Autodesk Inventor part; units mm, degrees
ref_plane "YZ Plane" through (0, 0, 0) normal (1, 0, 0) x (0, 1, 0)
ref_plane "XZ Plane" through (0, 0, 0) normal (0, 1, 0) x (-1, 0, 0)
ref_plane "XY Plane" through (0, 0, 0) normal (0, 0, 1) x (1, 0, 0)
sketch "Boceto1" plane through (0, 0, 0) normal (0, 1, 0) x (-1, 0, 0)
  line L0 (12.5, 6.25) -> (-12.5, 6.25)
  line L1 (-12.5, 6.25) -> (-12.5, -6.25)
  line L2 (-12.5, -6.25) -> (12.5, -6.25)
  line L3 (12.5, -6.25) -> (12.5, 6.25)
  line L4 (10.5, 4.25) -> (-10.5, 4.25)
  line L5 (-10.5, 4.25) -> (-10.5, -4.25)
  line L6 (-10.5, -4.25) -> (10.5, -4.25)
  line L7 (10.5, -4.25) -> (10.5, 4.25)
  point P0 (0, 0)
  point P1 (12.5, 0)
  point P2 (0, -6.25)
  point P3 (10.5, 0)
  point P4 (0, 4.25)
  dimension "d3" = 25
  dimension "d4" = 12.5
  dimension "d6" = 2
  dimension "d7" = 2
sketch "Boceto2" plane through (0, 0, 0) normal (0, 0, 1) x (1, 0, 0)
  line L0 (0, 0) -> (-62.7506, -84.1864)
  line L1 (0, 0) -> (0, -34.6116) construction
  dimension "d2" = 36.7
  dimension "d5" = 105
sweep "Barrido1" add profiles "Boceto1" path "Boceto2"
sketch "Boceto3" plane through (-12.5, 0, 6.25) normal (0, 0, 1) x (1, 0, 0)
  line L0 (0, 0) -> (25, 0)
  line L1 (0, 0) -> (-62.7506, -84.1864)
  line L2 (-37.7506, -84.1864) -> (-62.7506, -84.1864)
  line L3 (25, 0) -> (-37.7506, -84.1864)
  line L4 (25, 0) -> (-37.7506, -84.1864)
  line L5 (25, 0) -> (-36.551, -82.5769)
  line L6 (-37.7506, -84.1864) -> (-62.7506, -84.1864)
  line L7 (0, 0) -> (-62.7506, -84.1864)
  line L8 (-55.6056, -74.6007) -> (0, 0)
  line L9 (0, 0) -> (25, 0)
  line L10 (0, 0) -> (25, 0)
  line L11 (-39.7581, -84.1864) -> (-50.795, -84.1864)
  arc A0 (-39.7581, -84.1864) -> (-36.551, -82.5769) centre (-39.7581, -80.1864) ccw
  arc A1 (-55.6056, -74.6007) -> (-50.795, -84.1864) centre (-50.795, -78.1864) ccw
  line L12 (12.5, 0) -> (-50.2506, -84.1864)
  dimension "d10" = 4
  dimension "d11" = 6
extrude "Extrusión1" cut sketch "Boceto3" against normal blind 12 contours L0 L12 L2 A1 L1 | L0 L3 A0 L2 L12 keep common part
sketch "Boceto4" plane through (-12.5, 0, 6.25) normal (0, 0, 1) x (1, 0, 0)
  circle A0 centre (-42.6056, -74.1864) radius 5
  line L0 (-39.7581, -84.1864) -> (-50.795, -84.1864)
  line L1 (0, 0) -> (-55.6056, -74.6007)
  point P0 (12.5, 0)
  dimension "d16" = 10
  dimension "d17" = 13
  dimension "d18" = 10
extrude "Extrusión2" cut sketch "Boceto4" against normal blind 12
equation "\"d4\" = 0.5 * d3"
properties part number "Asiento - Soporte Manija" material "Aluminio 6061"
Check sheet for the modelled part. Datum: model origin and axes. Units: mm. A direction names the side the tool comes from. Give positions to 0.01 mm unless a question says otherwise; leave off trailing zeros. Write each loop counter-clockwise with the first axis right and the second up, starting at its lowest first coordinate (ties: lowest second). Pieces come first, ordered by that corner, then holes. Notation, with made-up numbers: (72.25, 22.5) -> (129.25, 22.5) arc R23 ccw to (129.25, 30.5) -> close; hole circle Ø1 at (69, 29). An arc over 180 degrees is marked (long way). Write item = value, one per line.
Item 1: Sectioned sample at B-B on y = -57.5. Record the boundary of the cut face in (x, z), and give its area (4 significant figures).
Output:
outline = (-55.36, -5.75) -> (-30.36, -5.75) -> (-30.36, 6.25) -> (-55.36, 6.25) -> close; hole (-53.36, -4.25) -> (-32.36, -4.25) -> (-32.36, 4.25) -> (-53.36, 4.25) -> close
area = 121.5 mm^2
Item 2: Release check for a two-part mould opening along Z. For faces 3 (the flat face through (-29, -39, -5.75)), 4 (the flat face through (-29, -39, 4.25)), 5 (the cylindrical face through (-56.19, -79.068, 5.264)) record: +Z half, -Z half, draft (parallel to the pull), parting line (faces both ways), or undercut.
Output:
face_3 = -Z half
face_4 = undercut
face_5 = draft
Item 3: Scan lines: probe 1 along Z at (x, y) = (-18.5, -26); probe 2 along X at (y, z) = (-9, -1); probe 3 along X at (y, z) = (-42, 3). Record each from-to range of solid material in increasing order. Write a range as from..to.
Output:
probe_1 = -5.75..-4.25, 4.25..6.25
probe_2 = -19.21..-17.21, 3.79..5.79
probe_3 = -43.81..-41.81, -20.81..-18.81
Item 4: Sectioned sample at C-C on z = -2.75. Record the boundary of the cut face in (x, y).
Output:
outline = (-69.26, -78.83) -> (-10.5, 0) -> (-12.5, 0) -> (-68.11, -74.6) arc R6 ccw to start; (-52.25, -84.19) arc R4 ccw to (-49.05, -82.58) -> (12.5, 0) -> (10.5, 0) -> close
Item 5: Gauge pin test, flat ends, axial feed: pin 1 (3 mm diameter, centred on y = -37.5, z = 4, fed in from -X); pin 2 (2 mm diameter, centred on x = -53, z = 2, fed in from +Y); pin 3 (5 mm diameter, centred on y = -39.5, z = 3.5, fed in from +X). Record the tip position at first contact, or that the pin passes through.
Output:
pin_1 = -41.57
pin_2 = -52.99
pin_3 = -15.08
Item 6: Tool access check on faces 1 (the cylindrical face through (-69.29, -77.94, 0.33)), 2 (the flat face through (-40.291, -39.968, 0.059)). Record the directions out of +Z, -Z, +X, -X, +Y, -Y that give a thin tool (end or side, any length) a straight path to the whole face; none if there is none.
Output:
face_1 = +Z, -Z, -X
face_2 = none
Item 7: Sectioned sample at A-A on z = 5.25. Record the boundary of the cut face in (x, y) (3 decimals).
Output:
outline = (-68.106, -74.601) arc R6 ccw to (-63.295, -84.186) -> (-52.258, -84.186) arc R4 ccw to (-49.051, -82.577) -> (12.5, 0) -> (-12.5, 0) -> close; hole circle Ø10 at (-55.106, -74.186)
Item 8: Sectioned sample at D-D on x = -34. Record the boundary of the cut face in (y, z).
Output:
outline = (-62.38, -5.75) -> (-28.84, -5.75) -> (-28.84, 6.25) -> (-62.38, 6.25) -> close; hole (-59.7, -4.25) -> (-31.53, -4.25) -> (-31.53, 4.25) -> (-59.7, 4.25) -> close
